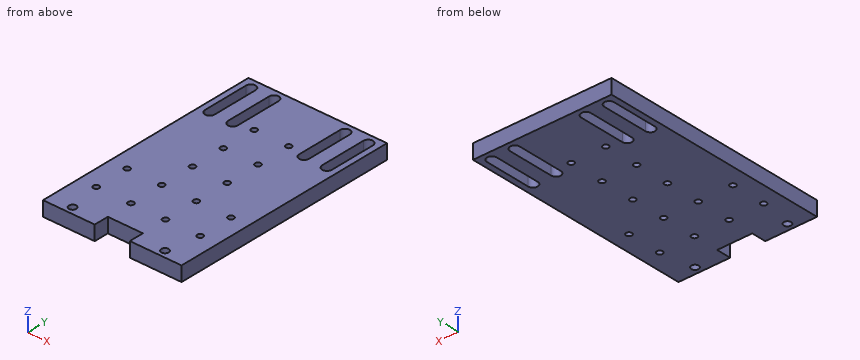
from build123d import *

# Parameters (mm, degrees)
BOSS_EXTRUDE1_DEPTH             = 6.35
F_2_5_2_5_DIAMETER_HOLE1_D      = 2.5
F_2_5_2_5_DIAMETER_HOLE1_DEPTH  = 6.35
F_3_2_3_2_DIAMETER_HOLE1_D      = 3.2
F_3_2_3_2_DIAMETER_HOLE1_DEPTH  = 6.35
F_2_5_2_5_DIAMETER_HOLE2_D      = 2.5
F_2_5_2_5_DIAMETER_HOLE2_DEPTH  = 6.35
F_2_5_2_5_DIAMETER_HOLE3_D      = 2.5
F_2_5_2_5_DIAMETER_HOLE3_DEPTH  = 6.35
F_2_5_2_5_DIAMETER_HOLE4_D      = 2.5
F_2_5_2_5_DIAMETER_HOLE4_DEPTH  = 6.35
F_2_5_2_5_DIAMETER_HOLE5_D      = 2.5
F_2_5_2_5_DIAMETER_HOLE5_DEPTH  = 6.35
F_2_5_2_5_DIAMETER_HOLE6_D      = 2.5
F_2_5_2_5_DIAMETER_HOLE6_DEPTH  = 6.35
F_2_5_2_5_DIAMETER_HOLE7_D      = 2.5
F_2_5_2_5_DIAMETER_HOLE7_DEPTH  = 6.35
F_2_5_2_5_DIAMETER_HOLE8_D      = 2.5
F_2_5_2_5_DIAMETER_HOLE8_DEPTH  = 6.35
F_2_5_2_5_DIAMETER_HOLE9_D      = 2.5
F_2_5_2_5_DIAMETER_HOLE9_DEPTH  = 6.35
F_2_5_2_5_DIAMETER_HOLE10_D     = 2.5
F_2_5_2_5_DIAMETER_HOLE10_DEPTH = 6.35
F_2_5_2_5_DIAMETER_HOLE11_D     = 2.5
F_2_5_2_5_DIAMETER_HOLE11_DEPTH = 6.35
F_2_5_2_5_DIAMETER_HOLE12_D     = 2.5
F_2_5_2_5_DIAMETER_HOLE12_DEPTH = 6.35
F_2_5_2_5_DIAMETER_HOLE13_D     = 2.5
F_2_5_2_5_DIAMETER_HOLE13_DEPTH = 6.35
F_2_5_2_5_DIAMETER_HOLE14_D     = 2.5
F_2_5_2_5_DIAMETER_HOLE14_DEPTH = 6.35
F_3_2_3_2_DIAMETER_HOLE2_D      = 3.2
F_3_2_3_2_DIAMETER_HOLE2_DEPTH  = 6.35
CUT_EXTRUDE1_DEPTH              = 7.35


with BuildPart() as part:
    # Sketch1 → Boss-Extrude1 (new body)
    with BuildSketch(Plane.XY.offset(118.288574318)):
        Polygon((19.634665341, 102.188959457), (19.634665341, 2.188959457), (42.034665341, 2.188959457), (42.034665341, 8.538959457), (57.234665341, 8.538959457), (57.234665341, 2.188959457), (79.634665341, 2.188959457), (79.634665341, 102.188959457), align=None)
    extrude(amount=-BOSS_EXTRUDE1_DEPTH)

    # Ø2.5 (2.5) Diameter Hole1
    with Locations(Plane(origin=(0, 0, 111.938574318), x_dir=(-1, 0, 0), z_dir=(0, 0, -1))):
        with Locations((-27.134665341, 19.688959457)):
            Hole(F_2_5_2_5_DIAMETER_HOLE1_D / 2, depth=F_2_5_2_5_DIAMETER_HOLE1_DEPTH)

    # Ø3.2 (3.2) Diameter Hole1
    with Locations(Plane.XY.offset(118.288574318)):
        with Locations((29.634665341, 5.363959457)):
            Hole(F_3_2_3_2_DIAMETER_HOLE1_D / 2, depth=F_3_2_3_2_DIAMETER_HOLE1_DEPTH)

    # Ø2.5 (2.5) Diameter Hole2
    with Locations(Plane(origin=(0, 0, 111.938574318), x_dir=(-1, 0, 0), z_dir=(0, 0, -1))):
        with Locations((-57.134665341, 19.688959457)):
            Hole(F_2_5_2_5_DIAMETER_HOLE2_D / 2, depth=F_2_5_2_5_DIAMETER_HOLE2_DEPTH)

    # Ø2.5 (2.5) Diameter Hole3
    with Locations(Plane(origin=(0, 0, 111.938574318), x_dir=(-1, 0, 0), z_dir=(0, 0, -1))):
        with Locations((-42.134665341, 34.688959457)):
            Hole(F_2_5_2_5_DIAMETER_HOLE3_D / 2, depth=F_2_5_2_5_DIAMETER_HOLE3_DEPTH)

    # Ø2.5 (2.5) Diameter Hole4
    with Locations(Plane(origin=(0, 0, 111.938574318), x_dir=(-1, 0, 0), z_dir=(0, 0, -1))):
        with Locations((-42.134665341, 64.688959457)):
            Hole(F_2_5_2_5_DIAMETER_HOLE4_D / 2, depth=F_2_5_2_5_DIAMETER_HOLE4_DEPTH)

    # Ø2.5 (2.5) Diameter Hole5
    with Locations(Plane(origin=(0, 0, 111.938574318), x_dir=(-1, 0, 0), z_dir=(0, 0, -1))):
        with Locations((-57.134665341, 64.688959457)):
            Hole(F_2_5_2_5_DIAMETER_HOLE5_D / 2, depth=F_2_5_2_5_DIAMETER_HOLE5_DEPTH)

    # Ø2.5 (2.5) Diameter Hole6
    with Locations(Plane(origin=(0, 0, 111.938574318), x_dir=(-1, 0, 0), z_dir=(0, 0, -1))):
        with Locations((-27.134665341, 34.688959457)):
            Hole(F_2_5_2_5_DIAMETER_HOLE6_D / 2, depth=F_2_5_2_5_DIAMETER_HOLE6_DEPTH)

    # Ø2.5 (2.5) Diameter Hole7
    with Locations(Plane(origin=(0, 0, 111.938574318), x_dir=(-1, 0, 0), z_dir=(0, 0, -1))):
        with Locations((-72.134665341, 19.688959457)):
            Hole(F_2_5_2_5_DIAMETER_HOLE7_D / 2, depth=F_2_5_2_5_DIAMETER_HOLE7_DEPTH)

    # Ø2.5 (2.5) Diameter Hole8
    with Locations(Plane(origin=(0, 0, 111.938574318), x_dir=(-1, 0, 0), z_dir=(0, 0, -1))):
        with Locations((-42.134665341, 19.688959457)):
            Hole(F_2_5_2_5_DIAMETER_HOLE8_D / 2, depth=F_2_5_2_5_DIAMETER_HOLE8_DEPTH)

    # Ø2.5 (2.5) Diameter Hole9
    with Locations(Plane(origin=(0, 0, 111.938574318), x_dir=(-1, 0, 0), z_dir=(0, 0, -1))):
        with Locations((-57.134665341, 34.688959457)):
            Hole(F_2_5_2_5_DIAMETER_HOLE9_D / 2, depth=F_2_5_2_5_DIAMETER_HOLE9_DEPTH)

    # Ø2.5 (2.5) Diameter Hole10
    with Locations(Plane(origin=(0, 0, 111.938574318), x_dir=(-1, 0, 0), z_dir=(0, 0, -1))):
        with Locations((-42.134665341, 49.688959457)):
            Hole(F_2_5_2_5_DIAMETER_HOLE10_D / 2, depth=F_2_5_2_5_DIAMETER_HOLE10_DEPTH)

    # Ø2.5 (2.5) Diameter Hole11
    with Locations(Plane(origin=(0, 0, 111.938574318), x_dir=(-1, 0, 0), z_dir=(0, 0, -1))):
        with Locations((-42.134665341, 79.688959457)):
            Hole(F_2_5_2_5_DIAMETER_HOLE11_D / 2, depth=F_2_5_2_5_DIAMETER_HOLE11_DEPTH)

    # Ø2.5 (2.5) Diameter Hole12
    with Locations(Plane(origin=(0, 0, 111.938574318), x_dir=(-1, 0, 0), z_dir=(0, 0, -1))):
        with Locations((-57.134665341, 79.688959457)):
            Hole(F_2_5_2_5_DIAMETER_HOLE12_D / 2, depth=F_2_5_2_5_DIAMETER_HOLE12_DEPTH)

    # Ø2.5 (2.5) Diameter Hole13
    with Locations(Plane(origin=(0, 0, 111.938574318), x_dir=(-1, 0, 0), z_dir=(0, 0, -1))):
        with Locations((-57.134665341, 49.688959457)):
            Hole(F_2_5_2_5_DIAMETER_HOLE13_D / 2, depth=F_2_5_2_5_DIAMETER_HOLE13_DEPTH)

    # Ø2.5 (2.5) Diameter Hole14
    with Locations(Plane(origin=(0, 0, 111.938574318), x_dir=(-1, 0, 0), z_dir=(0, 0, -1))):
        with Locations((-72.134665341, 34.688959457)):
            Hole(F_2_5_2_5_DIAMETER_HOLE14_D / 2, depth=F_2_5_2_5_DIAMETER_HOLE14_DEPTH)

    # Ø3.2 (3.2) Diameter Hole2
    with Locations(Plane.XY.offset(118.288574318)):
        with Locations((69.634665341, 5.363959457)):
            Hole(F_3_2_3_2_DIAMETER_HOLE2_D / 2, depth=F_3_2_3_2_DIAMETER_HOLE2_DEPTH)

    # Sketch38 → Cut-Extrude1 (cut, through all)
    with BuildSketch(Plane.XY.offset(118.288574318)):
        with BuildLine():
            Line((22.134665341, 98.188959457), (22.134665341, 78.188959457))
            ThreePointArc((22.134665341, 78.188959457), (24.234665341, 76.088959457), (26.334665341, 78.188959457))
            Line((26.334665341, 78.188959457), (26.334665341, 98.188959457))
            ThreePointArc((26.334665341, 98.188959457), (24.234665341, 100.288959457), (22.134665341, 98.188959457))
        make_face()
        with BuildLine():
            Line((32.134665341, 98.188959457), (32.134665341, 78.188959457))
            ThreePointArc((32.134665341, 78.188959457), (34.234665341, 76.088959457), (36.334665341, 78.188959457))
            Line((36.334665341, 78.188959457), (36.334665341, 98.188959457))
            ThreePointArc((36.334665341, 98.188959457), (34.234665341, 100.288959457), (32.134665341, 98.188959457))
        make_face()
        with BuildLine():
            Line((62.934665341, 98.188959457), (62.934665341, 78.188959457))
            ThreePointArc((62.934665341, 78.188959457), (65.034665341, 76.088959457), (67.134665341, 78.188959457))
            Line((67.134665341, 78.188959457), (67.134665341, 98.188959457))
            ThreePointArc((67.134665341, 98.188959457), (65.034665341, 100.288959457), (62.934665341, 98.188959457))
        make_face()
        with BuildLine():
            Line((72.934665341, 98.188959457), (72.934665341, 78.188959457))
            ThreePointArc((72.934665341, 78.188959457), (75.034665341, 76.088959457), (77.134665341, 78.188959457))
            Line((77.134665341, 78.188959457), (77.134665341, 98.188959457))
            ThreePointArc((77.134665341, 98.188959457), (75.034665341, 100.288959457), (72.934665341, 98.188959457))
        make_face()
    extrude(amount=-CUT_EXTRUDE1_DEPTH, mode=Mode.SUBTRACT)


solid = part.part
CAD build for the part. Positions are in the model's coordinates, mm. Coordinates: 2 decimals unless noted, no trailing zeros. Write each loop counter-clockwise with the first axis right and the second up, starting at its lowest first coordinate (ties: lowest second). Pieces come first, ordered by that corner, then holes. Notation, with made-up numbers: (37.5, 14.5) - (50.5, 14.5) arc R19 cw to (50.5, 44.5) - close; hole circle Ø4 at (8, 36.5). An arc over 180 degrees is marked (long way). Use a Markdown table: item, result. Add a question column.
Item 1: Band-saw the part on C-C, the plane x = 53.5. Give the cut face in (y, z), and give its area (3 significant figures).
Item 2: Band-saw the part on B-B, the plane x = 66. Give the cut face in (y, z).
Item 3: Band-saw the part on D-D, the plane z = 114. Give the number of separate pieces and of enclosed holes in the cut face, and give its area (3 significant figures).
Item 4: Flat gauge pin, fed straight in: pin 1 (1.9 mm diameter, centred on x = 48, z = 116, fed in from -Y). Where does the tip first touch, or does it go through?
Item 5: Band-saw the part on A-A, the plane y = 88.5. Give the cut face in (x, z), and give its area (3 significant figures).
Item 6: Drill centre lines: L1, parallel to Y at x = 72, z = 114.25; L2, parallel to X at y = 96, z = 114.5; L3, parallel to Y at x = 72.5, z = 112.25. Where is each one in solid material? Low to high. Write a range as from..to.
Numbers:
| question | item | result |
|---|---|---|
| 1 | outline | (8.54, 111.94) - (102.19, 111.94) - (102.19, 118.29) - (8.54, 118.29) - close |
| 1 | area | 595 mm2 |
| 2 | outline | (2.19, 111.94) - (76.32, 111.94) - (76.32, 118.29) - (2.19, 118.29) - close; (100.05, 111.94) - (102.19, 111.94) - (102.19, 118.29) - (100.05, 118.29) - close |
| 3 | separate pieces | 1 |
| 3 | enclosed holes | 20 |
| 3 | area | 5,430 mm2 |
| 4 | pin 1 | y = 8.54 |
| 5 | outline | (19.63, 111.94) - (22.13, 111.94) - (22.13, 118.29) - (19.63, 118.29) - close; (26.33, 111.94) - (32.13, 111.94) - (32.13, 118.29) - (26.33, 118.29) - close; (36.33, 111.94) - (62.93, 111.94) - (62.93, 118.29) - (36.33, 118.29) - close; (67.13, 111.94) - (72.93, 111.94) - (72.93, 118.29) - (67.13, 118.29) - close; (77.13, 111.94) - (79.63, 111.94) - (79.63, 118.29) - (77.13, 118.29) - close |
| 5 | area | 274 mm2 |
| 6 | L1 | 2.19..18.45, 20.93..33.45, 35.93..102.19 |
| 6 | L2 | 19.63..22.13, 26.33..32.13, 36.33..62.93, 67.13..72.93, 77.13..79.63 |
| 6 | L3 | 2.19..18.49, 20.88..33.49, 35.88..102.19 |
